```python
from build123d import *

# Parameters (mm, degrees)
BOSS_EXTRUDE1_DEPTH            = 1.6
F_2_2_2_2_DIAMETER_HOLE2_D     = 2.2
F_2_2_2_2_DIAMETER_HOLE1_D     = 2.2
F_2_2_2_2_DIAMETER_HOLE1_DEPTH = 2
SKETCH7_W                      = 0.2
SKETCH7_H                      = 100.7
EXTRUDE1_DEPTH                 = 2.6


with BuildPart() as part:
    # Sketch1 → Boss-Extrude1 (new body)
    with BuildSketch(Plane(origin=(0, 0, 0), x_dir=(1, 0, 0), z_dir=(0, 1, 0))):
        Polygon((65.24, 10.562547362), (65.24, -54.937452638), (65.24, -68.137452638), (-17.76, -68.137452638), (-17.76, -46.137452638), (-17.76, 19.362547362), (-17.76, 32.562547362), (65.24, 32.562547362), align=None)
    extrude(amount=BOSS_EXTRUDE1_DEPTH)

    # Ø2.2 (2.2) Diameter Hole2 (through all)
    with Locations(Plane(origin=(0, 1.6, 0), x_dir=(1, 0, 0), z_dir=(0, 1, 0))):
        with Locations((-0.76, 29.462547362), (48.24, 29.462547362)):
            Hole(F_2_2_2_2_DIAMETER_HOLE2_D / 2)

    # Ø2.2 (2.2) Diameter Hole1
    with Locations(Plane(origin=(0, 1.6, 0), x_dir=(1, 0, 0), z_dir=(0, 1, 0))):
        with Locations((-9.76, -64.537452638), (57.24, -64.537452638)):
            Hole(F_2_2_2_2_DIAMETER_HOLE1_D / 2, depth=F_2_2_2_2_DIAMETER_HOLE1_DEPTH)

    # Sketch7 → Extrude1 (cut, through all)
    with BuildSketch(Plane.XZ):
        with Locations((-17.66, 17.787452638)):
            Rectangle(SKETCH7_W, SKETCH7_H)
        with Locations((65.14, 17.787452638)):
            Rectangle(SKETCH7_W, SKETCH7_H)
    extrude(amount=-EXTRUDE1_DEPTH, mode=Mode.SUBTRACT)


solid = part.part
```
Here's how the part is built. I have some questions about the finished solid (model axes, mm). Give positions to 0.01 mm unless a question says otherwise; leave off trailing zeros. Write each loop counter-clockwise with the first axis right and the second up, starting at its lowest first coordinate (ties: lowest second). Pieces come first, ordered by that corner, then holes.
(1) Will this pin go through, and if not, where does the flat tip stop? pin 1 (3 mm diameter, centred on x = 57.24, z = 64.54, fed in from +Y).
Output values:
pin 1: stops at y = 1.6
(2) Thinking about a two-plate mould opening in Z: for faces 1 (the face through (24, 1.6, 17)), 2 (the face through (56.19, 0.79, 64.21)), 3 (the face through (-10.776, 0.789, 64.959)), which applies, pulls with the +Z half, pulls with the -Z half, needs draft (parallel to the pull), parting line crosses it, or undercut?
Output values:
face 1: needs draft
face 2: undercut
face 3: undercut
(3) Imagine slicing it at A-A, the plane x = -0.76. Write out the boundary of the cut face in (y, z), and give its area (3 significant figures).
Output values:
outline: (0, -32.56) - (1.6, -32.56) - (1.6, -30.56) - (0, -30.56) - close; (0, -28.36) - (1.6, -28.36) - (1.6, 68.14) - (0, 68.14) - close
area: 158 mm2
(4) If I drill on L1, parallel to Z at x = -9.76, y = 1.2; L2, parallel to Z at x = 48, y = 0.2, over which ranges is the centre line in solid material (lowest first)?
Output values:
L1: z = -32.56 to 63.44, 65.64 to 68.14
L2: z = -32.56 to -30.54, -28.39 to 68.14
